Part model, mm, in its own coordinate system. Face numbers are marked on the shaded views. A direction names the side the tool comes from. Coordinates: 2 decimals unless noted, no trailing zeros. Write each loop counter-clockwise with the first axis right and the second up, starting at its lowest first coordinate (ties: lowest second). Pieces come first, ordered by that corner, then holes. Notation, with made-up numbers: (-3.75, 73.25) -> (47.25, 73.25) arc R16 cw to (47.25, 97.25) -> close; hole circle Ø6 at (15, -28.75). An arc over 180 degrees is marked (long way). Write item = value, one per line.
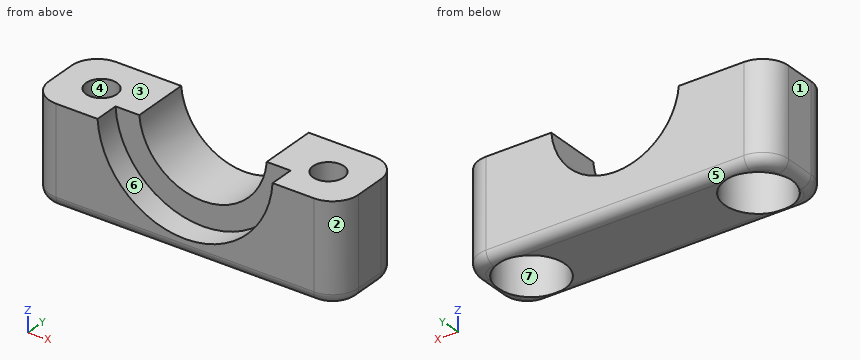
from build123d import *

# Parameters (mm, degrees)
F0_W         = 30
F0_H         = 8
F0_R         = 1.5
F1_DEPTH     = 10
F2_R         = 3.25
F2_R_2       = 1.5
F3_DEPTH     = 4
F5_DEPTH     = 8.001
F7_DEPTH     = 2.4
F8_R         = 2.5
F9_T1_DEPTH  = 3
F9_T3_DEPTH  = 25
F9_T6_ANGLE  = 90
F9_T8_ANGLE  = 90
F9_T10_ANGLE = 90
F9_T12_ANGLE = 90
F10_W        = 35.437501967
F10_H        = 11.6335232742
F10_R        = 1.5
F11_DEPTH    = 0.5


# Not quite as in the source:
# - a fillet or chamfer that OpenCascade refuses, or shapes differently, is made with other operations: its cross-section is extruded or revolved along the edge and cut away or added


with BuildPart() as f1:
    # F0 (on Top) → F1 (new body)
    with BuildSketch(Plane.XY):
        Rectangle(F0_W, F0_H)
        with Locations((-11, 0)):
            Circle(F0_R, mode=Mode.SUBTRACT)
        with Locations((11, 0)):
            Circle(F0_R, mode=Mode.SUBTRACT)
    extrude(amount=F1_DEPTH)

    # F2 (on face) → F3 (cut)
    with BuildSketch(Plane(origin=(0, 0, 0), x_dir=(1, 0, 0), z_dir=(0, 0, -1))):
        with Locations((11, 0)):
            Circle(F2_R)
        with Locations((11, 0)):
            Circle(F2_R_2, mode=Mode.SUBTRACT)
        with Locations((-11, 0)):
            Circle(F2_R)
        with Locations((-11, 0)):
            Circle(F2_R_2, mode=Mode.SUBTRACT)
    extrude(amount=-F3_DEPTH, mode=Mode.SUBTRACT)

    # F4 (on face) → F5 (cut, through all)
    with BuildSketch(Plane(origin=(0, 4, 0), x_dir=(-1, 0, 0), z_dir=(0, 1, 0))):
        with BuildLine():
            ThreePointArc((-6.2, 10), (0, 3.8), (6.2, 10))
            Line((6.2, 10), (-6.2, 10))
        make_face()
    extrude(amount=-F5_DEPTH, mode=Mode.SUBTRACT)

    # F6 (on face) → F7 (cut)
    with BuildSketch(Plane.XZ.offset(4)):
        with BuildLine():
            ThreePointArc((-8.5, 10), (0, 1.5), (8.5, 10))
            Line((8.5, 10), (6.2, 10))
            ThreePointArc((6.2, 10), (0, 3.8), (-6.2, 10))
            Line((-6.2, 10), (-8.5, 10))
        make_face()
    extrude(amount=-F7_DEPTH, mode=Mode.SUBTRACT)

    # F8
    f8_edges = [f1.edges().sort_by_distance(p)[0] for p in [
        (15, 4, 5),
        (15, -4, 5),
        (-15, 4, 5),
        (-15, -4, 5),
    ]]
    fillet(f8_edges, radius=F8_R)

    # F9: fillet of radius 1 on 8 edges, made by hand

    # F9_s2 → F9_t1 (cut)
    with BuildSketch(Plane.XZ.offset(-1.5)):
        with BuildLine():
            ThreePointArc((14, 0), (14.7071067812, 0.2928932188), (15, 1))
            Line((15, 1), (15, 0))
            Line((15, 0), (14, 0))
        make_face()
        with BuildLine():
            ThreePointArc((-14, 0), (-14.7071067812, 0.2928932188), (-15, 1))
            Line((-15, 1), (-15, 0))
            Line((-15, 0), (-14, 0))
        make_face()
    extrude(amount=F9_T1_DEPTH, mode=Mode.SUBTRACT)

    # F9_s4 → F9_t3 (cut)
    with BuildSketch(Plane.YZ.offset(-12.5)):
        with BuildLine():
            ThreePointArc((4, 1), (3.7071067812, 0.2928932188), (3, 0))
            Line((3, 0), (4, 0))
            Line((4, 0), (4, 1))
        make_face()
        with BuildLine():
            ThreePointArc((-3, 0), (-3.7071067812, 0.2928932188), (-4, 1))
            Line((-4, 1), (-4, 0))
            Line((-4, 0), (-3, 0))
        make_face()
    extrude(amount=F9_T3_DEPTH, mode=Mode.SUBTRACT)

    # F9_s5 → F9_t6 (revolve, cut)
    with BuildSketch(Plane.YZ.offset(12.5)):
        with BuildLine():
            ThreePointArc((3, 0), (3.7071067812, 0.2928932188), (4, 1))
            Line((4, 1), (4, 0))
            Line((4, 0), (3, 0))
        make_face()
    revolve(axis=Axis((12.5, 1.5, 0), (0, 0, -1)), revolution_arc=F9_T6_ANGLE, mode=Mode.SUBTRACT)

    # F9_s7 → F9_t8 (revolve, cut)
    with BuildSketch(Plane.YZ.offset(-12.5)):
        with BuildLine():
            ThreePointArc((3, 0), (3.7071067812, 0.2928932188), (4, 1))
            Line((4, 1), (4, 0))
            Line((4, 0), (3, 0))
        make_face()
    revolve(axis=Axis((-12.5, 1.5, 0), (0, 0, 1)), revolution_arc=F9_T8_ANGLE, mode=Mode.SUBTRACT)

    # F9_s9 → F9_t10 (revolve, cut)
    with BuildSketch(Plane.XZ.offset(1.5)):
        with BuildLine():
            ThreePointArc((14, 0), (14.7071067812, 0.2928932188), (15, 1))
            Line((15, 1), (15, 0))
            Line((15, 0), (14, 0))
        make_face()
    revolve(axis=Axis((12.5, -1.5, 0), (0, 0, -1)), revolution_arc=F9_T10_ANGLE, mode=Mode.SUBTRACT)

    # F9_s11 → F9_t12 (revolve, cut)
    with BuildSketch(Plane.XZ.offset(1.5)):
        with BuildLine():
            ThreePointArc((-14, 0), (-14.7071067812, 0.2928932188), (-15, 1))
            Line((-15, 1), (-15, 0))
            Line((-15, 0), (-14, 0))
        make_face()
    revolve(axis=Axis((-12.5, -1.5, 0), (0, 0, 1)), revolution_arc=F9_T12_ANGLE, mode=Mode.SUBTRACT)

    # F10 (on face) → F11 (cut)
    with BuildSketch(Plane.XY.offset(10)):
        with Locations((0.726422295, -0.4176155198)):
            Rectangle(F10_W, F10_H)
        with BuildLine():
            Line((12.5, -4), (8.5, -4))
            Line((8.5, -4), (8.5, -1.6))
            Line((8.5, -1.6), (6.2, -1.6))
            Line((6.2, -1.6), (6.2, 4))
            Line((6.2, 4), (12.5, 4))
            ThreePointArc((12.5, 4), (14.267766953, 3.267766953), (15, 1.5))
            Line((15, 1.5), (15, -1.5))
            ThreePointArc((15, -1.5), (14.267766953, -3.267766953), (12.5, -4))
        make_face(mode=Mode.SUBTRACT)
        with BuildLine():
            Line((8.5, -1.6), (8.5, -4))
            Line((8.5, -4), (12.5, -4))
            ThreePointArc((12.5, -4), (14.267766953, -3.267766953), (15, -1.5))
            Line((15, -1.5), (15, 1.5))
            ThreePointArc((15, 1.5), (14.267766953, 3.267766953), (12.5, 4))
            Line((12.5, 4), (6.2, 4))
            Line((6.2, 4), (6.2, -1.6))
            Line((6.2, -1.6), (8.5, -1.6))
        make_face()
        with Locations((11, 0)):
            Circle(F10_R, mode=Mode.SUBTRACT)
    extrude(amount=-F11_DEPTH, mode=Mode.SUBTRACT)


solid = f1.part
Q1. Mould opens along X. For the marked faces 1, 2, 3 and 4 say: released by +X, released by -X, zero draft, split by the parting line, or undercut.
Model answer:
face_1 = released by -X
face_2 = released by +X
face_3 = zero draft
face_4 = undercut
Q2. Saw through at B-B on x = -11. Give the cut face in (y, z), and give its area (3 significant figures).
Model answer:
outline = (-4, 1) arc R1 ccw to (-3.25, 0.03) -> (-3.25, 4) -> (-1.5, 4) -> (-1.5, 9.5) -> (-4, 9.5) -> close; (1.5, 4) -> (3.25, 4) -> (3.25, 0.03) arc R1 ccw to (4, 1) -> (4, 9.5) -> (1.5, 9.5) -> close
area = 33.1 mm²
Q3. Saw through at C-C on z = 2.5. Give the cut face in (x, y).
Model answer:
outline = (-15, -1.5) arc R2.5 ccw to (-12.5, -4) -> (-4, -4) -> (-4, -1.6) -> (4, -1.6) -> (4, -4) -> (12.5, -4) arc R2.5 ccw to (15, -1.5) -> (15, 1.5) arc R2.5 ccw to (12.5, 4) -> (-12.5, 4) arc R2.5 ccw to (-15, 1.5) -> close; hole circle Ø6.5 at (-11, 0); hole circle Ø6.5 at (11, 0)
Q4. Pin check, flat tips, straight feed: pin 1 (4 mm diameter, centred on x = 3, z = 6, fed in from -Y); pin 2 (3 mm diameter, centred on x = -11.5, y = -0.5, fed in from -Z). Stop position of each tip, or through.
Model answer:
pin_1 = -1.6
pin_2 = 4
Q5. Saw through at A-A on z = 9. Give the cut face in (x, y).
Model answer:
outline = (-15, -1.5) arc R2.5 ccw to (-12.5, -4) -> (-8.44, -4) -> (-8.44, -1.6) -> (-6.12, -1.6) -> (-6.12, 4) -> (-12.5, 4) arc R2.5 ccw to (-15, 1.5) -> close; (6.12, -1.6) -> (8.44, -1.6) -> (8.44, -4) -> (12.5, -4) arc R2.5 ccw to (15, -1.5) -> (15, 1.5) arc R2.5 ccw to (12.5, 4) -> (6.12, 4) -> close; hole circle Ø3 at (-11, 0); hole circle Ø3 at (11, 0)
Q6. Probe line 1 (X direction, y = 0, z = 3); line 2 (Y direction, x = 11, z = 2.9); line 3 (X direction, y = 2, z = 1.25). List the from-to ranges inside material, lowest first. Write a range as from..to.
Model answer:
line_1 = -15..-14.25, -7.75..7.75, 14.25..15
line_2 = -4..-3.25, 3.25..4
line_3 = -14.95..-13.56, -8.44..8.44, 13.56..14.95
Q7. Saw through at D-D on y = 0. Give the cut face in (x, z).
Model answer:
outline = (-15, 1) arc R1 ccw to (-14.25, 0.03) -> (-14.25, 4) -> (-12.5, 4) -> (-12.5, 9.5) -> (-15, 9.5) -> close; (-9.5, 4) -> (-7.75, 4) -> (-7.75, 0) -> (7.75, 0) -> (7.75, 4) -> (9.5, 4) -> (9.5, 9.5) -> (6.18, 9.5) arc R6.2 cw to (-6.18, 9.5) -> (-9.5, 9.5) -> close; (12.5, 4) -> (14.25, 4) -> (14.25, 0.03) arc R1 ccw to (15, 1) -> (15, 9.5) -> (12.5, 9.5) -> close
Q8. Which spindle directions (+Z, -Z, +X, -X, +Y, -Y) get a long thin tool onto all of the face, cutting with end or side? Do the marked faces 5, 6 and 7. Say none if no direction does.
Model answer:
face_5 = -Z, +X, -X, +Y
face_6 = +Z, -Y
face_7 = -Z
